Autodesk Inventor part; units mm, degrees
ref_plane "nut_XY" through (0, 0, 0) normal (1, 0, 0) x (0, 0, -1)
ref_plane "nut_YZ" through (0, 0, 0) normal (0, 0, -1) x (0, 1, 0)
ref_plane "nut_ZX" through (0, 0, 0) normal (0, 1, 0) x (1, 0, 0)
sketch "Sketch_1" plane through (0, 0, 0) normal (0, 0, 1) x (1, 0, 0)
  arc A0 (-9, -4.5858) -> (-8.7071, -5.2929) centre (-8, -4.5858) ccw
  line L0 (-8.7071, -5.2929) -> (-5.7929, -8.2071)
  arc A1 (-5.7929, -8.2071) -> (-5.0858, -8.5) centre (-5.0858, -7.5) ccw
  line L1 (-5.0858, -8.5) -> (-4, -8.5)
  arc A2 (-4, -8.5) -> (-3, -7.5) centre (-4, -7.5) ccw
  line L2 (-3, -7.5) -> (-3, -4.9)
  line L3 (-3, -4.9) -> (0, -4.9)
  line L4 (0, -4.9) -> (0, 4.9)
  line L5 (0, 4.9) -> (-3, 4.9)
  line L6 (-3, 4.9) -> (-3, 7.5)
  arc A3 (-3, 7.5) -> (-4, 8.5) centre (-4, 7.5) ccw
  line L7 (-4, 8.5) -> (-5.0858, 8.5)
  arc A4 (-5.0858, 8.5) -> (-5.7929, 8.2071) centre (-5.0858, 7.5) ccw
  line L8 (-5.7929, 8.2071) -> (-8.7071, 5.2929)
  arc A5 (-8.7071, 5.2929) -> (-9, 4.5858) centre (-8, 4.5858) ccw
  line L9 (-9, 4.5858) -> (-9, -4.5858)
extrude "Extrusion1" add sketch "Sketch_1" along normal mid plane 17
sketch "Sketch_5" plane through (0, 0, 0) normal (0, 0, 1) x (1, 0, 0)
  line L0 (0, 0) -> (-9, 0)
  line L1 (-9, 0) -> (-9, 4)
  line L2 (-9, 4) -> (-8.3235, 3.3235)
  line L3 (-8.3235, 3.3235) -> (-0.6765, 3.3235)
  line L4 (-0.6765, 3.3235) -> (0, 4)
  line L5 (0, 4) -> (0, 0)
  line L6 (0, 0) -> (-9, 0)
revolve "Revolution1" cut sketch "Sketch_5" angle 360 about axis through (0, 0, 0) along (1, 0, 0)
thread "Thread1"
ref_plane "nut_XY" through (0, 0, 0) normal (1, 0, 0) x (0, 0, -1)
ref_plane "nut_YZ" through (0, 0, 0) normal (0, 0, -1) x (0, 1, 0)
ref_plane "nut_ZX" through (0, 0, 0) normal (0, 1, 0) x (1, 0, 0)
ref_plane "to_bolt_XY" through (-9, 0, 0) normal (1, 0, 0) x (0, 0, -1)
ref_plane "to_bolt_YZ" through (-9, 0, 0) normal (0, 0, -1) x (0, 1, 0)
ref_plane "to_bolt_ZX" through (-9, 0, 0) normal (0, 1, 0) x (1, 0, 0)
ref_plane "to_frames_XY" through (-3, 0, 0) normal (1, 0, 0) x (0, 0, -1)
ref_plane "to_frames_YZ" through (-3, 0, 0) normal (0, 0, -1) x (0, 1, 0)
ref_plane "to_frames_ZX" through (-3, 0, 0) normal (0, 1, 0) x (1, 0, 0)
properties part number "HNTT8-8"
Input: part model. Units: mm. Frame: model coordinates. A direction names the side the tool comes from. Coordinates: 2 decimals unless noted, no trailing zeros. Loops run counter-clockwise (first coordinate to the right, second up) from the corner with the lowest first, then second, coordinate; pieces in that order, holes last.
Q1. Set-up query: faces 1 (the flat face through (-1, 4.9, 0)), 2 (the flat face through (-5, 0, -8.5)), 3 (the flat face through (-2, -4.9, 0)). Return all of +Z, -Z, +X, -X, +Y, -Y with unobstructed straight access to the full face (end or side cutting, diameter ignored); none if empty.
Results are:
face 1: +Z, -Z, +X, +Y
face 2: -Z, +X, -X, +Y, -Y
face 3: +Z, -Z, +X, -Y
Q2. Section C-C, the plane x = -4.25. Return the cut outline in (y, z), and give its area (3 significant figures).
Results are:
outline: (-8.5, -8.5) - (8.5, -8.5) - (8.5, 8.5) - (-8.5, 8.5) - close; hole circle Ø6.65 at (0, 0)
area: 254 mm2
Q3. Mould query, pull axis Y, two halves, no side actions, for faces 4 (the cylindrical face through (-3.285, -8.199, -0.119)), 5 (the flat face through (-3, 6, 0)), 6 (the flat face through (-4.5, 8.5, -0.1)), 7 (the cylindrical face through (-4.45, 3.07, -1.27)). Classes: +Y half, -Y half, draft (parallel to the pull), parting line (faces both ways), or undercut.
Results are:
face 4: -Y half
face 5: draft
face 6: +Y half
face 7: undercut
Q4. Contact query for flat-ended pins moving along their axis: pin 1 (2.5 mm diameter, centred on x = -2, z = -3.5, fed in from +Y); pin 2 (1 mm diameter, centred on x = -7.5, z = 3.5, fed in from -Y); pin 3 (3 mm diameter, centred on y = -6.5, z = 5, fed in from -X). Output: stop coordinate, or through.
Results are:
pin 1: stops at y = 8.16
pin 2: stops at y = -7
pin 3: stops at x = -8.91
Q5. Section D-D, the plane z = -5.5. Return the cut outline in (x, y).
Results are:
outline: (-9, -4.59) arc R1 ccw to (-8.71, -5.29) - (-5.79, -8.21) arc R1 ccw to (-5.09, -8.5) - (-4, -8.5) arc R1 ccw to (-3, -7.5) - (-3, -4.9) - (0, -4.9) - (0, 4.9) - (-3, 4.9) - (-3, 7.5) arc R1 ccw to (-4, 8.5) - (-5.09, 8.5) arc R1 ccw to (-5.79, 8.21) - (-8.71, 5.29) arc R1 ccw to (-9, 4.59) - close
Q6. Section B-B, the plane y = 0. Return the cut outline in (x, z).
Results are:
outline: (-9, -8.5) - (0, -8.5) - (0, -4) - (-0.68, -3.32) - (-8.32, -3.32) - (-9, -4) - close; (-9, 4) - (-8.32, 3.32) - (-0.68, 3.32) - (0, 4) - (0, 8.5) - (-9, 8.5) - close
Q7. Section A-A, the plane z = 0. Return the cut outline in (x, y).
Results are:
outline: (-9, -4.59) arc R1 ccw to (-8.71, -5.29) - (-5.79, -8.21) arc R1 ccw to (-5.09, -8.5) - (-4, -8.5) arc R1 ccw to (-3, -7.5) - (-3, -4.9) - (0, -4.9) - (0, -4) - (-0.68, -3.32) - (-8.32, -3.32) - (-9, -4) - close; (-9, 4) - (-8.32, 3.32) - (-0.68, 3.32) - (0, 4) - (0, 4.9) - (-3, 4.9) - (-3, 7.5) arc R1 ccw to (-4, 8.5) - (-5.09, 8.5) arc R1 ccw to (-5.79, 8.21) - (-8.71, 5.29) arc R1 ccw to (-9, 4.59) - close
Q8. Line query: line 1 along Z through (x, y) = (-2.25, 0); line 2 along X through (y, z) = (-6.5, -1.5); line 3 along Y through (x, z) = (-2, -7.25). Output: solid intervals per line, ascending.
Results are:
line 1: z = -8.5 to -3.32, 3.32 to 8.5
line 2: x = -7.5 to -3
line 3: y = -4.9 to 4.9
